```python
from build123d import *

# Parameters (mm, degrees)
SKETCH1_W                    = 50.8
SKETCH1_H                    = 25.4
BOSS_EXTRUDE1_DEPTH          = 44.45
SKETCH8_W                    = 13.97
SKETCH8_H                    = 19.685
SKETCH8_W_2                  = 22.86
SKETCH8_W_3                  = 38.1
SKETCH8_H_2                  = 15.875
CUT_EXTRUDE1_DEPTH           = 58.15
F_8_CLEARANCE_HOLE3_D        = 4.4958
F_8_CLEARANCE_HOLE2_D        = 4.4958
F_1_8_0_18_DOWEL_HOLE1_D     = 4.572
F_1_8_0_18_DOWEL_HOLE1_DEPTH = 7.62
F_1_8_0_18_DOWEL_HOLE1_TIP   = 1.373567375
FILLET1_R                    = 2.54
SKETCH17_R                   = 1.27
CUT_EXTRUDE3_DEPTH           = 12.7


with BuildPart() as part:
    # Sketch1 → Boss-Extrude1 (new body)
    with BuildSketch(Plane(origin=(0, 0, 0), x_dir=(1, 0, 0), z_dir=(0, 1, 0))):
        Rectangle(SKETCH1_W, SKETCH1_H)
    extrude(amount=BOSS_EXTRUDE1_DEPTH)

    # Sketch8 → Cut-Extrude1 (cut, through all)
    with BuildSketch(Plane.XY.offset(12.7)):
        with Locations((-18.415, 9.8425)):
            Rectangle(SKETCH8_W, SKETCH8_H)
        with Locations((0, 9.8425)):
            Rectangle(SKETCH8_W_2, SKETCH8_H)
        with Locations((0, 36.5125)):
            Rectangle(SKETCH8_W_3, SKETCH8_H_2)
    extrude(amount=-CUT_EXTRUDE1_DEPTH, mode=Mode.SUBTRACT)

    # #8 Clearance Hole3 (through all)
    with Locations(Plane(origin=(25.4, 0, 0), x_dir=(0, 0, -1), z_dir=(1, 0, 0))):
        with Locations((6.868185943, 36.83), (-5.831814057, 36.83)):
            Hole(F_8_CLEARANCE_HOLE3_D / 2)

    # #8 Clearance Hole2 (through all)
    with Locations(Plane(origin=(0, 28.575, 0), x_dir=(1, 0, 0), z_dir=(0, 1, 0))):
        with Locations((0, 8.255), (0, -8.255)):
            Hole(F_8_CLEARANCE_HOLE2_D / 2)

    # 1/8 (0.18) Dowel Hole1
    with Locations(Plane.ZY.offset(-11.43)):
        with Locations((2.916276039, 6.096)):
            Hole(F_1_8_0_18_DOWEL_HOLE1_D / 2, depth=F_1_8_0_18_DOWEL_HOLE1_DEPTH)
            with Locations((0, 0, -(F_1_8_0_18_DOWEL_HOLE1_DEPTH + F_1_8_0_18_DOWEL_HOLE1_TIP / 2))):  # 118° drill point
                Cone(0, F_1_8_0_18_DOWEL_HOLE1_D / 2, F_1_8_0_18_DOWEL_HOLE1_TIP, mode=Mode.SUBTRACT)

    # Fillet1
    fillet1_edges = [part.edges().sort_by_distance(p)[0] for p in [
        (11.43, 19.685, 0),
        (19.05, 28.575, 0),
        (-19.05, 28.575, 0),
    ]]
    fillet(fillet1_edges, radius=FILLET1_R)

    # Sketch17 → Cut-Extrude3 (cut)
    with BuildSketch(Plane.XY.offset(-12.7)):
        with Locations((-22.225, 27.508501284)):
            Circle(SKETCH17_R)
        with Locations((22.225, 27.508501284)):
            Circle(SKETCH17_R)
    extrude(amount=CUT_EXTRUDE3_DEPTH, mode=Mode.SUBTRACT)


solid = part.part
```
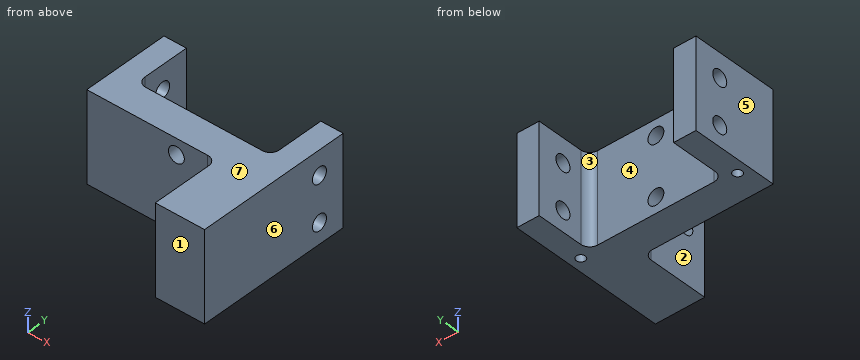
CAD build for the part. Positions are in the model's coordinates, mm. Face numbers are marked on the shaded views. A direction names the side the tool comes from. Give positions to 0.01 mm unless a question says otherwise; leave off trailing zeros. Write each loop counter-clockwise with the first axis right and the second up, starting at its lowest first coordinate (ties: lowest second). Pieces come first, ordered by that corner, then holes. Notation, with made-up numbers: M 16.25,28.5 L 42.25,28.5 A27 ccw 42.25,57.5 Z; hole C 43.5,-16.5 d1. An arc over 180 degrees is marked long. Return JSON: item names as keys, results as strings. Group by question number.
(1) Band-saw the part on A-A (x = 0). Give the cut face in (y, z) (3 decimals).
(2) Band-saw the part on C-C (x = 18). Give the cut face in (y, z), and give its area (3 significant figures).
(3) Flat gauge pins, fed straight in: pin 1 Ø4 at (y, z) = (36.83, 5.83) entering from -X; pin 2 Ø7 at (x, z) = (0, -8.255) entering from +Y (3 decimals); pin 3 Ø8 at (x, z) = (-15.5, -1) entering from -Y (3 decimals). Where does each tip first touch, or does it go through?
(4) Band-saw the part on D-D (y = 16.5). Give the cut face in (x, z).
(5) Band-saw the part on B-B (y = 36.83). Give the cut face in (x, z).
(6) Mould opens along X. For the marked faces 4, 5, 6 and 7 say: pulls with the +X half, pulls with the -X half, needs draft (parallel to the pull), parting line crosses it, or undercut.
(7) Drill centre lines: L1, parallel to X at y = 38, z = -9; L2, parallel to X at y = 27, z = -6.5; L3, parallel to X at y = 4.5, z = -9.75. Where is each one in solid material? Low to high. Write a range as [from, to].
(8) 3-axis set-ups, long thin cutter, end or side, ignore diameter. For the marked faces 1, 2 and 3: which of +Z, -Z, +X, -X, +Y, -Y reach the whole face in a straight line?
Entries:
{
 "1": {"outline": "M 19.685,-12.7 L 28.575,-12.7 L 28.575,-10.503 L 19.685,-10.503 Z; M 19.685,-6.007 L 28.575,-6.007 L 28.575,6.007 L 19.685,6.007 Z; M 19.685,10.503 L 28.575,10.503 L 28.575,12.7 L 19.685,12.7 Z"},
 "2": {"outline": "M 0,-12.7 L 29.06,-12.7 L 29.06,12.7 L 0,12.7 Z; hole C 6.1,2.92 d4.57", "area": "722 mm^2"},
 "3": {"pin 1": "passes through", "pin 2": "stops at y = 28.575", "pin 3": "stops at y = 19.685"},
 "4": {"outline": "M 11.43,-12.7 L 25.4,-12.7 L 25.4,12.7 L 11.43,12.7 Z"},
 "5": {"outline": "M -25.4,-12.7 L -19.05,-12.7 L -19.05,-9.12 L -25.4,-9.12 Z; M -25.4,-4.62 L -19.05,-4.62 L -19.05,3.58 L -25.4,3.58 Z; M -25.4,8.08 L -19.05,8.08 L -19.05,12.7 L -25.4,12.7 Z; M 19.05,-12.7 L 25.4,-12.7 L 25.4,-9.12 L 19.05,-9.12 Z; M 19.05,-4.62 L 25.4,-4.62 L 25.4,3.58 L 19.05,3.58 Z; M 19.05,8.08 L 25.4,8.08 L 25.4,12.7 L 19.05,12.7 Z"},
 "6": {"face 4": "undercut", "face 5": "pulls with the -X half", "face 6": "pulls with the +X half", "face 7": "needs draft"},
 "7": {"L1": "x = [-25.4, -19.05], [19.05, 25.4]", "L2": "x = [-25.4, -23.39], [-21.06, -1.4], [1.4, 21.06], [23.39, 25.4]", "L3": "x = [11.43, 25.4]"},
 "8": {"face 1": "+Z, -Z, +X, -X, -Y", "face 2": "+Z, -Z, -X, -Y", "face 3": "+Z, -Z, +Y"}
}
